Design review of the part built by this model. Coordinates are the model's own, in mm. Face numbers are marked on the shaded views. A direction names the side the tool comes from. Give positions to 0.01 mm unless a question says otherwise; leave off trailing zeros. Loops run counter-clockwise (first coordinate to the right, second up) from the corner with the lowest first, then second, coordinate; pieces in that order, holes last. Notation, with made-up numbers: (88, 39.25) -> (98, 39.25) arc R30 ccw to (98, 78.25) -> close; hole circle Ø1 at (-39, -21). An arc over 180 degrees is marked (long way). Use a Markdown table: item, result. Add a question column.
1. To check wall thickness, follow line 1 (Z direction, x = -3.5, y = -0.25); line 2 (Y direction, x = -1.5, z = 34); line 3 (Y direction, x = -0.5, z = 23). State the ranges of each line that lie inside material, in increasing order.
2. For pin 1 Ø1.9 at (y, z) = (0.5, 39) entering from -X (3 decimals); pin 2 Ø1 at (x, z) = (-0.5, 29) entering from +Y; pin 3 Ø1.5 at (x, z) = (-2.5, 5) entering from -Y; pin 4 Ø1.5 at (y, z) = (-1, 20.5) entering from -X, all flat-tipped, find the tip position at first contact; note any pin that passes through.
3. For the marked faces 1 and 2, list the 3-axis set-ups (+Z, -Z, +X, -X, +Y, -Y) from which the entire face can be reached by the end or side of a thin tool; tool diameter is ignored.
4. Add section B-B (z = 5.5). State the section outline as (x, y) points.
5. Add section A-A (z = 20). State the section outline as (x, y) points.
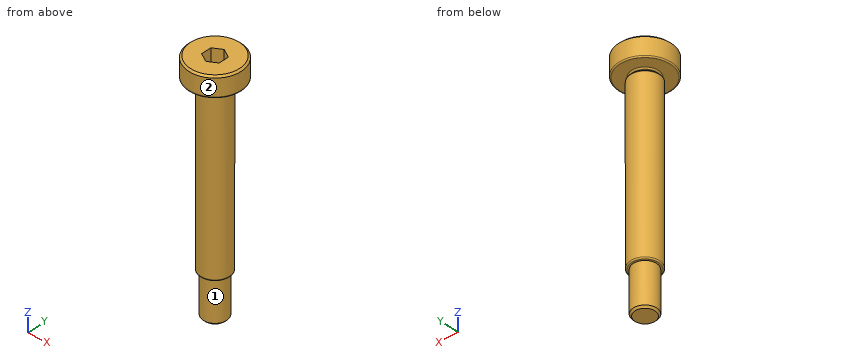
Solid Edge part; units mm, degrees
sketch "Sketch1" plane through (0, 0, 0) normal (0, -1, 0) x (1, 0, 0)
  line L0 (0, 40.7) -> (4.505, 40.7)
  line L1 (4.505, 40.7) -> (4.505, 37.25)
  line L2 (4.505, 37.25) -> (2.1, 37.25)
  line L3 (2.1, 37.25) -> (2.1, 36.85)
  line L4 (2.1, 36.85) -> (2.5, 36.85)
  line L5 (2.5, 36.85) -> (2.5, 7.25)
  line L6 (2.5, 7.25) -> (2, 7.25)
  line L7 (2, 7.25) -> (2, 0)
  line L8 (2, 0) -> (0, 0)
  dimension "D1" = 4.505
  dimension "D2" = 2.1
  dimension "D3" = 2
  dimension "D4" = 2.5
  dimension "D5" = 2
revolve "RevolvedProtrusion1" add sketch "Sketch1" angle 360 about axis through (0, 0, 0) along (0, 0, 1)
chamfer "Chamfer1" distance 0.3 angle 45 3 edges at (-2.5, 0, 36.85) (-4.505, 0, 40.7) (-2, 0, 0)
fillet "Round_1" radius 0.2 4 edges at (-4.505, 0, 37.25) (-2.1, 0, 37.25) (-2.5, 0, 7.25) (-2.5, 0, 36.55)
sketch "Sketch2" plane through (0, 0, 40.7) normal (0, 0, 1) x (1, 0, 0)
  line L0 (1.5, 0.866) -> (0, 1.7321)
  line L1 (0, 1.7321) -> (-1.5, 0.866)
  line L2 (-1.5, 0.866) -> (-1.5, -0.866)
  line L3 (-1.5, -0.866) -> (0, -1.7321)
  line L4 (0, -1.7321) -> (1.5, -0.866)
  line L5 (1.5, -0.866) -> (1.5, 0.866)
extrude "ExtrudedCutout_1" cut sketch "Sketch2" against normal blind 2.4
properties material "Stainless Steel, 304"
Taken from the geometry:
| question | item | result |
|---|---|---|
| 1 | line 1 | z = 37.25 to 40.7 |
| 1 | line 2 | y = -2 to 2 |
| 1 | line 3 | y = -2.45 to 2.45 |
| 2 | pin 1 | stops at x = -4.505 |
| 2 | pin 2 | stops at y = 2.5 |
| 2 | pin 3 | stops at y = -0.97 |
| 2 | pin 4 | stops at x = -2.49 |
| 3 | face 1 | -Z |
| 3 | face 2 | +Z, -Z |
| 4 | outline | circle Ø4 at (0, 0) |
| 5 | outline | circle Ø5 at (0, 0) |
